The listing builds one solid part. Answer for the finished solid, in the listing's coordinates (mm). Coordinates: 2 decimals unless noted, no trailing zeros. Order: outer loops, then holes, each group sorted by start corner. A loop starts at its lowest first (then second) coordinate and runs counter-clockwise, first axis right, second up. Notation, with made-up numbers: (26.25, 48.5) -> (83.25, 48.5) arc R13 ccw to (83.25, 66.5) -> close; hole circle Ø5 at (17, -27). An arc over 180 degrees is marked (long way). Write each question's results on one line, items separated by ' | '. Start each with the question number.
(1) The part is cut by section B-B, the plane x = 2.7. Give the vertices of the cut face in (y, z).
(2) Given pin 1 (3.5 mm diameter, centred on y = -231.5, z = 21, fed in from -X), flat-ended and moving along its own axis, determine where the tip first touches the part or whether it passes through.
(3) The part is cut by section A-A, the plane z = 43. Give the vertices of the cut face in (x, y) (3 decimals), then the cut area to 3 significant figures.
(4) The part is cut by section C-C, the plane y = -141. Give the vertices of the cut face in (x, z).
(5) Straight lines are drawn through the part: L1, parallel to Y at x = 0.45, z = 31; L2, parallel to Y at x = 2.45, z = 23.5; L3, parallel to Y at x = 2.5, z = 2. For each, find the intervals that lie inside material, in ascending order.
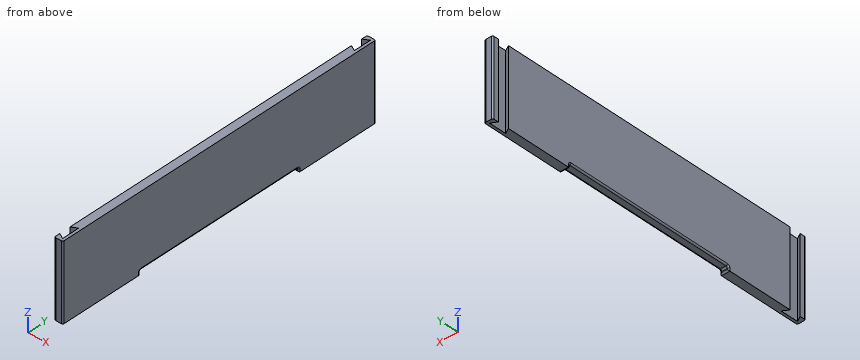
```python
from build123d import *

# Parameters (mm, degrees)
BOSS_EXTRUDE1_DEPTH = 53
CUT_EXTRUDE1_DEPTH  = 52
FILLET1_R           = 1
FILLET2_R           = 1


with BuildPart() as part:
    # Sketch2 → Boss-Extrude1 (new body)
    with BuildSketch(Plane.XY):
        Polygon((0, 0), (0, -4.14), (4.00969762, -1.825), (4.00969762, -14.175), (0, -11.86), (0, -19), (0, -219), (0, -226.14), (4.00969762, -223.825), (4.00969762, -236.175), (0, -233.86), (0, -238), (5.9, -238), (5.9, -229.334408546), (5.9, -8.665591454), (5.9, 0), align=None)
    extrude(amount=BOSS_EXTRUDE1_DEPTH)

    # Sketch3 → Cut-Extrude1 (cut)
    with BuildSketch(Plane(origin=(0, 0, 0), x_dir=(0, 0, -1), z_dir=(1, 0, 0))):
        Polygon((0, -119), (0, -58.5), (-2.8, -58.5), (-2.8, -179.5), (0, -179.5), align=None)
    extrude(amount=CUT_EXTRUDE1_DEPTH, mode=Mode.SUBTRACT)

    # Fillet1
    fillet1_edges = [part.edges().sort_by_distance(p)[0] for p in [
        (2.95, -179.5, 0),
        (2.95, -58.5, 0),
        (5.9, -119, 2.8),
        (2.95, -58.5, 2.8),
        (0, -119, 2.8),
        (0, -58.5, 1.4),
        (2.95, -179.5, 2.8),
        (0, -179.5, 1.4),
        (5.9, -58.5, 1.4),
        (5.9, -179.5, 1.4),
    ]]
    fillet(fillet1_edges, radius=FILLET1_R)

    # Fillet2
    fillet2_edges = [part.edges().sort_by_distance(p)[0] for p in [
        (5.9, 0, 26.5),
        (5.9, -238, 26.5),
        (0, -238, 26.5),
        (0, 0, 26.5),
    ]]
    fillet(fillet2_edges, radius=FILLET2_R)


solid = part.part
```
Established:
1) outline: (-238, 0) -> (-235.42, 0) -> (-235.42, 53) -> (-238, 53) -> close; (-224.58, 0) -> (-180.5, 0) arc R1 ccw to (-179.5, 1) -> (-179.5, 1.8) arc R1 cw to (-178.5, 2.8) -> (-59.5, 2.8) arc R1 cw to (-58.5, 1.8) -> (-58.5, 1) arc R1 ccw to (-57.5, 0) -> (-13.42, 0) -> (-13.42, 53) -> (-224.58, 53) -> close; (-2.58, 0) -> (0, 0) -> (0, 53) -> (-2.58, 53) -> close
2) pin 1: stops at x = 4.01
3) outline: (0, -237) arc R1 ccw to (1, -238) -> (4.9, -238) arc R1 ccw to (5.9, -237) -> (5.9, -1) arc R1 ccw to (4.9, 0) -> (1, 0) arc R1 ccw to (0, -1) -> (0, -4.14) -> (4.01, -1.825) -> (4.01, -14.175) -> (0, -11.86) -> (0, -226.14) -> (4.01, -223.825) -> (4.01, -236.175) -> (0, -233.86) -> close | area: 1,320 mm^2
4) outline: (0, 3.8) arc R1 ccw to (1, 2.8) -> (4.9, 2.8) arc R1 ccw to (5.9, 3.8) -> (5.9, 53) -> (0, 53) -> close
5) L1: y = -237.84 to -234.12, -225.88 to -12.12, -3.88 to -0.16 | L2: y = -238 to -235.27, -224.73 to -13.27, -2.73 to 0 | L3: y = -238 to -235.3, -224.7 to -179.48, -58.52 to -13.3, -2.7 to 0
